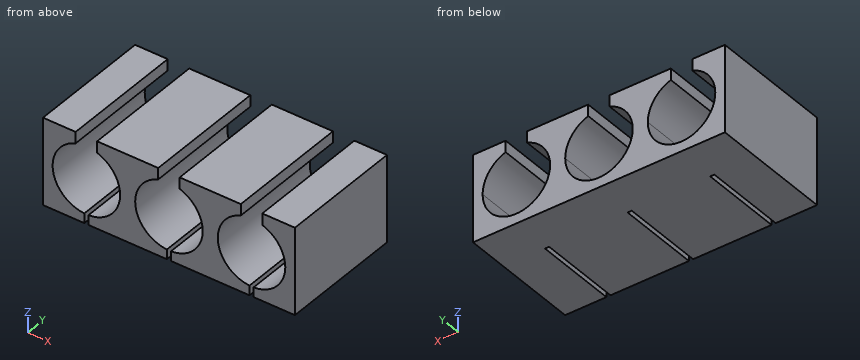
```python
from build123d import *

# Parameters (mm, degrees)
F1_DEPTH = 30
F3_W     = 1
F3_H     = 2.340305
F4_DEPTH = 20


with BuildPart() as f1:
    # F0 (on Front) → F1 (new body)
    with BuildSketch(Plane.XZ):
        with BuildLine():
            Line((-39.669828, 23.200569), (-47.569828, 23.200569))
            Line((-47.569828, 23.200569), (-47.569828, 2.200569))
            Line((-47.569828, 2.200569), (13.430172, 2.200569))
            Line((13.430172, 2.200569), (13.430172, 23.200569))
            Line((13.430172, 23.200569), (5.530172, 23.200569))
            Line((5.530172, 23.200569), (5.530172, 20.451093))
            ThreePointArc((5.530172, 20.451093), (9.566648, 17.474227), (11.105172, 12.700569))
            ThreePointArc((11.105172, 12.700569), (-1.843486, 6.064093), (0.330172, 20.451093))
            Line((0.330172, 20.451093), (0.330172, 23.200569))
            Line((0.330172, 23.200569), (-14.469828, 23.200569))
            Line((-14.469828, 23.200569), (-14.469828, 20.451093))
            ThreePointArc((-14.469828, 20.451093), (-10.433352, 17.474227), (-8.894828, 12.700569))
            ThreePointArc((-8.894828, 12.700569), (-21.843486, 6.064093), (-19.669828, 20.451093))
            Line((-19.669828, 20.451093), (-19.669828, 23.200569))
            Line((-19.669828, 23.200569), (-34.469828, 23.200569))
            Line((-34.469828, 23.200569), (-34.469828, 20.451093))
            ThreePointArc((-34.469828, 20.451093), (-30.433352, 17.474227), (-28.894828, 12.700569))
            ThreePointArc((-28.894828, 12.700569), (-41.843486, 6.064093), (-39.669828, 20.451093))
            Line((-39.669828, 20.451093), (-39.669828, 23.200569))
        make_face()
    extrude(amount=F1_DEPTH)

    # F3 (on face) → F4 (cut)
    with BuildSketch(Plane.XZ.offset(30)):
        with Locations((-37.069828, 3.370721)):
            Rectangle(F3_W, F3_H)
        with Locations((-17.069828, 3.370721)):
            Rectangle(F3_W, F3_H)
        with Locations((2.930172, 3.370721)):
            Rectangle(F3_W, F3_H)
    extrude(amount=-F4_DEPTH, mode=Mode.SUBTRACT)


solid = f1.part
```
Part model, mm, in its own coordinate system. Coordinates: 2 decimals unless noted, no trailing zeros. Loops run counter-clockwise (first coordinate to the right, second up) from the corner with the lowest first, then second, coordinate; pieces in that order, holes last. Notation, with made-up numbers: (56.25, -36.5) - (89.25, -36.5) arc R15 cw to (89.25, -8.5) - close; hole circle Ø8 at (-27.75, -22.5). An arc over 180 degrees is marked (long way). Write item = value, one per line. Start each with the question number.
Item 1: Cut at A-A, the plane y = -12.75. Give the cut face in (x, z) (3 decimals).
Item 2: Cut at C-C, the plane y = -8.5. Give the cut face in (x, z) (3 decimals).
Item 3: Wall check: L1, parallel to X at y = -23.75, z = 21; L2, parallel to X at y = -23, z = 4; L3, parallel to Z at x = -2.5, y = -18. Give the ranges that are in metal, low to high. Write a range as from..to.
Item 4: Cut at B-B, the plane z = 6. Give the cut face in (x, y), and give its area (3 significant figures).
Item 5: Flat gauge pins, fed straight in: pin 1 Ø1.5 at (x, y) = (-19, -22) entering from +Z; pin 2 Ø0.8 at (x, z) = (-37, 3.5) entering from -Y. Where does each tip first touch, or does it go through?
Item 6: Cut at D-D, the plane x = -4. Give the cut face in (y, z).
The answers:
q1.outline = (-47.57, 2.201) - (-37.57, 2.201) - (-37.57, 4.541) arc R8.175 cw to (-39.67, 20.451) - (-39.67, 23.201) - (-47.57, 23.201) - close; (-36.57, 2.201) - (-17.57, 2.201) - (-17.57, 4.541) arc R8.175 cw to (-19.67, 20.451) - (-19.67, 23.201) - (-34.47, 23.201) - (-34.47, 20.451) arc R8.175 cw to (-36.57, 4.541) - close; (-16.57, 2.201) - (2.43, 2.201) - (2.43, 4.541) arc R8.175 cw to (0.33, 20.451) - (0.33, 23.201) - (-14.47, 23.201) - (-14.47, 20.451) arc R8.175 cw to (-16.57, 4.541) - close; (3.43, 2.201) - (13.43, 2.201) - (13.43, 23.201) - (5.53, 23.201) - (5.53, 20.451) arc R8.175 cw to (3.43, 4.541) - close
q2.outline = (-47.57, 2.201) - (13.43, 2.201) - (13.43, 23.201) - (5.53, 23.201) - (5.53, 20.451) arc R8.175 cw (long way) to (0.33, 20.451) - (0.33, 23.201) - (-14.47, 23.201) - (-14.47, 20.451) arc R8.175 cw (long way) to (-19.67, 20.451) - (-19.67, 23.201) - (-34.47, 23.201) - (-34.47, 20.451) arc R8.175 cw (long way) to (-39.67, 20.451) - (-39.67, 23.201) - (-47.57, 23.201) - close
q3.L1 = -47.57..-39.67, -34.47..-19.67, -14.47..0.33, 5.53..13.43
q3.L2 = -47.57..-37.57, -36.57..-17.57, -16.57..2.43, 3.43..13.43
q3.L3 = 2.2..6.59, 18.81..23.2
q4.outline = (-47.57, -30) - (-41.75, -30) - (-41.75, 0) - (-47.57, 0) - close; (-32.39, -30) - (-21.75, -30) - (-21.75, 0) - (-32.39, 0) - close; (-12.39, -30) - (-1.75, -30) - (-1.75, 0) - (-12.39, 0) - close; (7.61, -30) - (13.43, -30) - (13.43, 0) - (7.61, 0) - close
q4.area = 987 mm2
q5.pin_1 = 23.2
q5.pin_2 = -10
q6.outline = (-30, 2.2) - (0, 2.2) - (0, 8.36) - (-30, 8.36) - close; (-30, 17.04) - (0, 17.04) - (0, 23.2) - (-30, 23.2) - close
